The listing builds one solid part. Answer for the finished solid, in the listing's coordinates (mm). A direction names the side the tool comes from. Round coordinates to 2 decimals unless told otherwise and drop trailing zeros. Loops run counter-clockwise (first coordinate to the right, second up) from the corner with the lowest first, then second, coordinate; pieces in that order, holes last. Notation, with made-up numbers: M 43,44 L 51,44 A20 ccw 51,67 Z; hole C 36,85 d2. An arc over 180 degrees is marked long. Put each result on its own line as item: value. Start each with the question number.
(1) Section B-B, the plane x = 3.75 is taken. Count the separate pieces of the cut face and the enclosed holes in it, then the cut area to 3 significant figures.
(2) Section C-C, the plane y = 10 is taken. Determine the outline of the cut face in (x, z) (3 decimals), then the cut area to 3 significant figures.
(3) Straight lines are drawn through the part: line 1 (Z direction, x = 7.25, y = 1.25); line 2 (X direction, y = 2, z = 6.5); line 3 (X direction, y = 8.75, z = -7). For each, find the intervals that lie inside material, in ascending order.
(4) Section D-D, the plane z = 17 is taken. Determine the outline of the cut face in (x, y).
(5) Determine the mould class of faces 3 (the face through (-1, 1.9, 23.8)), 4 (the face through (-2, 12.7, -3)), 5 (the face through (-7, 2.1, -28.8)) for opening direction Z: released by +Z, released by -Z, zero draft, split by the parting line, or undercut.
(6) Which of the six approach directions +Z, -Z, +X, -X, +Y, -Y give full straight-line access (tool end or side, diameter ignored) to faces 1 (the face through (0.117, 1.932, -23.993)), 2 (the face through (-5.334, 1.878, 0.016))?
(7) Section A-A, the plane z = 0 is taken. Determine the outline of the cut face in (x, y) (3 decimals), then the cut area to 3 significant figures.
(8) Flat-ended cylindrical pins translate along their axes: P1, Ø6, axis at x = -4.91, z = -4.91, coming from the -Y side; P2, Ø7, axis at x = -4.91, z = 4.91, coming from the +Y side; P3, Ø8, axis at x = 4, z = 20.5, coming from the +Y side; P4, Ø8, axis at x = 3.5, z = -27.5, coming from the +Y side. Find the tip coordinate at first contact, or state that the pin passes through.
```python
from build123d import *

# Parameters (mm, degrees)
SKETCH1_W               = 20
SKETCH1_H               = 63.5
BOSS_EXTRUDE1_DEPTH     = 12.7
SKETCH2_R               = 3.175
SKETCH2_R_2             = 2.1844
CUT_EXTRUDE1_DEPTH      = 36.62797356
CUT_EXTRUDE2_DEPTH      = 36.62797356
CUT_EXTRUDE2_DEPTH_BACK = 36.62797356
SKETCH4_R               = 3.81
CUT_EXTRUDE3_DEPTH      = 8.89
SKETCH4_3_R             = 3.81
SKETCH4_3_R_2           = 2.1844
SKETCH4_3_R_3           = 5.334
SKETCH4_3_R_4           = 3.175
CUT_EXTRUDE4_DEPTH      = 3.81
SKETCH6_R               = 5.08
SKETCH6_R_2             = 2.667
CUT_EXTRUDE5_DEPTH      = 8.89
SKETCH6_4_R             = 2.667
CUT_EXTRUDE6_DEPTH      = 35.454239272
FILLET1_R               = 10.16


with BuildPart() as part:
    # Sketch1 → Boss-Extrude1 (new body)
    with BuildSketch(Plane(origin=(0, 0, 0), x_dir=(1, 0, 0), z_dir=(0, 1, 0))):
        Rectangle(SKETCH1_W, SKETCH1_H)
    extrude(amount=BOSS_EXTRUDE1_DEPTH)

    # Sketch2 → Cut-Extrude1 (cut, through all)
    with BuildSketch(Plane(origin=(0, 12.7, 0), x_dir=(1, 0, 0), z_dir=(0, 1, 0))):
        with Locations(Location((0, 0, 0), (0, 0, 270))):
            Circle(SKETCH2_R)
        with Locations(Location((-4.912200098, 4.912200098, 0), (0, 0, 270))):
            Circle(SKETCH2_R_2)
        with Locations(Location((4.912200098, -4.912200098, 0), (0, 0, 270))):
            Circle(SKETCH2_R_2)
        with Locations(Location((4.912200098, 4.912200098, 0), (0, 0, 90))):
            Circle(SKETCH2_R_2)
        with Locations(Location((-4.912200098, -4.912200098, 0), (0, 0, 90))):
            Circle(SKETCH2_R_2)
    extrude(amount=-CUT_EXTRUDE1_DEPTH, mode=Mode.SUBTRACT)

    # Sketch3 → Cut-Extrude2 (cut, two sides: drawn at the far end of the back side and taken through both)
    with BuildSketch(Plane(origin=(0, 0, 0), x_dir=(0, 0, -1), z_dir=(1, 0, 0)).offset(-CUT_EXTRUDE2_DEPTH_BACK)):
        with BuildLine():
            Line((31.75, 3.81), (31.75, 12.7))
            Line((31.75, 12.7), (10.906600098, 12.7))
            ThreePointArc((10.906600098, 12.7), (16.898665682, 6.209564949), (25.4, 3.81))
            Line((25.4, 3.81), (31.75, 3.81))
        make_face()
        with BuildLine():
            ThreePointArc((-25.4, 3.81), (-16.898665682, 6.209564949), (-10.906600098, 12.7))
            Line((-10.906600098, 12.7), (-31.75, 12.7))
            Line((-31.75, 12.7), (-31.75, 3.81))
            Line((-31.75, 3.81), (-25.4, 3.81))
        make_face()
    extrude(amount=CUT_EXTRUDE2_DEPTH + CUT_EXTRUDE2_DEPTH_BACK, mode=Mode.SUBTRACT)

    # Sketch4 → Cut-Extrude3 (cut)
    with BuildSketch(Plane.XZ):
        with Locations((-4.912200098, -4.912200098)):
            Circle(SKETCH4_R)
        with Locations((4.912200098, 4.912200098)):
            Circle(SKETCH4_R)
        with Locations((-4.912200098, 4.912200098)):
            Circle(SKETCH4_R)
        with Locations((4.912200098, -4.912200098)):
            Circle(SKETCH4_R)
    extrude(amount=-CUT_EXTRUDE3_DEPTH, mode=Mode.SUBTRACT)

    # Sketch4<3> → Cut-Extrude4 (cut)
    # profile 1 of 28: a face of its own
    with BuildSketch(Plane.XZ):
        with Locations((-4.912200098, 4.912200098)):
            Circle(SKETCH4_3_R)
        with Locations(Location((-4.912200098, 4.912200098, 0), (0, 0, 270))):
            Circle(SKETCH4_3_R_2, mode=Mode.SUBTRACT)
    # profile 2 of 28: a face of its own
    with BuildSketch(Plane.XZ):
        Circle(SKETCH4_3_R_3)
        with Locations(Location((0, 0, 0), (0, 0, 90))):
            Circle(SKETCH4_3_R_4, mode=Mode.SUBTRACT)
    # profile 3 of 28: a face of its own
    with BuildSketch(Plane.XZ):
        Circle(SKETCH4_3_R_3)
    # profile 4 of 28: a face of its own
    with BuildSketch(Plane.XZ):
        with Locations(Location((-4.912200098, 4.912200098, 0), (0, 0, 270))):
            Circle(SKETCH4_3_R_2)
    # profile 5 of 28: a face of its own
    with BuildSketch(Plane.XZ):
        with Locations((-4.912200098, 4.912200098)):
            Circle(SKETCH4_3_R)
    # profile 6 of 28: a face of its own
    with BuildSketch(Plane.XZ):
        Circle(SKETCH4_3_R_3)
        with Locations(Location((0, 0, 0), (0, 0, 90))):
            Circle(SKETCH4_3_R_4, mode=Mode.SUBTRACT)
    # profile 7 of 28: a face of its own
    with BuildSketch(Plane.XZ):
        with Locations((-4.912200098, -4.912200098)):
            Circle(SKETCH4_3_R)
    # profile 8 of 28: a face of its own
    with BuildSketch(Plane.XZ):
        Circle(SKETCH4_3_R_3)
        with Locations(Location((0, 0, 0), (0, 0, 90))):
            Circle(SKETCH4_3_R_4, mode=Mode.SUBTRACT)
    # profile 9 of 28: a face of its own
    with BuildSketch(Plane.XZ):
        with Locations((-4.912200098, -4.912200098)):
            Circle(SKETCH4_3_R)
        with Locations(Location((-4.912200098, -4.912200098, 0), (0, 0, 90))):
            Circle(SKETCH4_3_R_2, mode=Mode.SUBTRACT)
    # profile 10 of 28: a face of its own
    with BuildSketch(Plane.XZ):
        Circle(SKETCH4_3_R_3)
    # profile 11 of 28: a face of its own
    with BuildSketch(Plane.XZ):
        with Locations(Location((-4.912200098, -4.912200098, 0), (0, 0, 90))):
            Circle(SKETCH4_3_R_2)
    # profile 12 of 28: a face of its own
    with BuildSketch(Plane.XZ):
        with BuildLine():
            ThreePointArc((1.973854475, -2.486870224), (1.04518229, -2.998035854), (0, -3.175))
            Line((0, -3.175), (0, -5.334))
            ThreePointArc((0, -5.334), (0.560277089, -5.304492962), (1.114355409, -5.216298306))
            ThreePointArc((1.114355409, -5.216298306), (1.278123958, -3.767826643), (1.973854475, -2.486870224))
        make_face()
    # profile 13 of 28: a face of its own
    with BuildSketch(Plane.XZ):
        with BuildLine():
            Line((0, -5.334), (0, -3.175))
            ThreePointArc((0, -3.175), (-1.04518229, -2.998035854), (-1.973854475, -2.486870224))
            ThreePointArc((-1.973854475, -2.486870224), (-1.326729639, -3.623595587), (-1.102200098, -4.912200098))
            ThreePointArc((-1.102200098, -4.912200098), (-1.105240139, -5.064370621), (-1.114355409, -5.216298306))
            ThreePointArc((-1.114355409, -5.216298306), (-0.560277089, -5.304492962), (0, -5.334))
        make_face()
    # profile 14 of 28: a face of its own
    with BuildSketch(Plane.XZ):
        with Locations((4.912200098, -4.912200098)):
            Circle(SKETCH4_3_R)
        with Locations(Location((4.912200098, -4.912200098, 0), (0, 0, 270))):
            Circle(SKETCH4_3_R_2, mode=Mode.SUBTRACT)
    # profile 15 of 28: a face of its own
    with BuildSketch(Plane.XZ):
        Circle(SKETCH4_3_R_3)
        with Locations(Location((0, 0, 0), (0, 0, 90))):
            Circle(SKETCH4_3_R_4, mode=Mode.SUBTRACT)
    # profile 16 of 28: a face of its own
    with BuildSketch(Plane.XZ):
        Circle(SKETCH4_3_R_3)
    # profile 17 of 28: a face of its own
    with BuildSketch(Plane.XZ):
        with Locations(Location((4.912200098, -4.912200098, 0), (0, 0, 270))):
            Circle(SKETCH4_3_R_2)
    # profile 18 of 28: a face of its own
    with BuildSketch(Plane.XZ):
        with Locations((4.912200098, -4.912200098)):
            Circle(SKETCH4_3_R)
    # profile 19 of 28: a face of its own
    with BuildSketch(Plane.XZ):
        Circle(SKETCH4_3_R_3)
        with Locations(Location((0, 0, 0), (0, 0, 90))):
            Circle(SKETCH4_3_R_4, mode=Mode.SUBTRACT)
    # profile 20 of 28: a face of its own
    with BuildSketch(Plane.XZ):
        with Locations((4.912200098, 4.912200098)):
            Circle(SKETCH4_3_R)
    # profile 21 of 28: a face of its own
    with BuildSketch(Plane.XZ):
        Circle(SKETCH4_3_R_3)
        with Locations(Location((0, 0, 0), (0, 0, 90))):
            Circle(SKETCH4_3_R_4, mode=Mode.SUBTRACT)
    # profile 22 of 28: a face of its own
    with BuildSketch(Plane.XZ):
        with Locations((4.912200098, 4.912200098)):
            Circle(SKETCH4_3_R)
        with Locations(Location((4.912200098, 4.912200098, 0), (0, 0, 90))):
            Circle(SKETCH4_3_R_2, mode=Mode.SUBTRACT)
    # profile 23 of 28: a face of its own
    with BuildSketch(Plane.XZ):
        Circle(SKETCH4_3_R_3)
    # profile 24 of 28: a face of its own
    with BuildSketch(Plane.XZ):
        with Locations(Location((4.912200098, 4.912200098, 0), (0, 0, 90))):
            Circle(SKETCH4_3_R_2)
    # profile 25 of 28: a face of its own
    with BuildSketch(Plane.XZ):
        with BuildLine():
            Line((0, 3.175), (0, 5.334))
            ThreePointArc((0, 5.334), (-0.560277089, 5.304492962), (-1.114355409, 5.216298306))
            ThreePointArc((-1.114355409, 5.216298306), (-1.105240139, 5.064370621), (-1.102200098, 4.912200098))
            ThreePointArc((-1.102200098, 4.912200098), (-1.326729639, 3.623595587), (-1.973854475, 2.486870224))
            ThreePointArc((-1.973854475, 2.486870224), (-1.04518229, 2.998035854), (0, 3.175))
        make_face()
    # profile 26 of 28: a face of its own
    with BuildSketch(Plane.XZ):
        with BuildLine():
            ThreePointArc((1.114355409, 5.216298306), (0.560277089, 5.304492962), (0, 5.334))
            Line((0, 5.334), (0, 3.175))
            ThreePointArc((0, 3.175), (1.04518229, 2.998035854), (1.973854475, 2.486870224))
            ThreePointArc((1.973854475, 2.486870224), (1.278123958, 3.767826643), (1.114355409, 5.216298306))
        make_face()
    # profile 27 of 28: a face of its own
    with BuildSketch(Plane.XZ):
        with BuildLine():
            ThreePointArc((1.973854475, 2.486870224), (1.04518229, 2.998035854), (0, 3.175))
            Line((0, 3.175), (0, -3.175))
            ThreePointArc((0, -3.175), (1.04518229, -2.998035854), (1.973854475, -2.486870224))
            ThreePointArc((1.973854475, -2.486870224), (2.218123262, -2.218123262), (2.486870224, -1.973854475))
            ThreePointArc((2.486870224, -1.973854475), (2.998035854, -1.04518229), (3.175, 0))
            ThreePointArc((3.175, 0), (2.998035854, 1.04518229), (2.486870224, 1.973854475))
            ThreePointArc((2.486870224, 1.973854475), (2.218123262, 2.218123262), (1.973854475, 2.486870224))
        make_face()
    # profile 28 of 28: a face of its own
    with BuildSketch(Plane.XZ):
        with BuildLine():
            Line((0, -3.175), (0, 3.175))
            ThreePointArc((0, 3.175), (-1.04518229, 2.998035854), (-1.973854475, 2.486870224))
            ThreePointArc((-1.973854475, 2.486870224), (-2.218123262, 2.218123262), (-2.486870224, 1.973854475))
            ThreePointArc((-2.486870224, 1.973854475), (-3.175, 0), (-2.486870224, -1.973854475))
            ThreePointArc((-2.486870224, -1.973854475), (-2.218123262, -2.218123262), (-1.973854475, -2.486870224))
            ThreePointArc((-1.973854475, -2.486870224), (-1.04518229, -2.998035854), (0, -3.175))
        make_face()
    extrude(amount=-CUT_EXTRUDE4_DEPTH, mode=Mode.SUBTRACT)

    # Sketch6 → Cut-Extrude5 (cut)
    # profile 1 of 3: a face of its own
    with BuildSketch(Plane(origin=(0, 3.81, 0), x_dir=(1, 0, 0), z_dir=(0, 1, 0))):
        with Locations((0, -21.328300049)):
            Circle(SKETCH6_R)
        with Locations((0, -21.328300049)):
            Circle(SKETCH6_R_2, mode=Mode.SUBTRACT)
    # profile 2 of 3: a face of its own
    with BuildSketch(Plane(origin=(0, 3.81, 0), x_dir=(1, 0, 0), z_dir=(0, 1, 0))):
        with Locations((0, -21.328300049)):
            Circle(SKETCH6_R_2)
    # profile 3 of 3: a face of its own
    with BuildSketch(Plane(origin=(0, 3.81, 0), x_dir=(1, 0, 0), z_dir=(0, 1, 0))):
        with Locations((0, 21.328300049)):
            Circle(SKETCH6_R)
    extrude(amount=CUT_EXTRUDE5_DEPTH, mode=Mode.SUBTRACT)

    # Sketch6<4> → Cut-Extrude6 (cut, through all)
    with BuildSketch(Plane(origin=(0, 3.81, 0), x_dir=(1, 0, 0), z_dir=(0, 1, 0))):
        with Locations(Location((0, 21.328300049, 0), (0, 0, 270))):
            Circle(SKETCH6_4_R)
        with Locations(Location((0, -21.328300049, 0), (0, 0, 270))):
            Circle(SKETCH6_4_R)
    extrude(amount=-CUT_EXTRUDE6_DEPTH, mode=Mode.SUBTRACT)

    # Fillet1
    # the kernel refuses this fillet: 10.16 mm, written as the material it takes off along each edge
    with BuildSketch(Plane(origin=(10, -25.4, 31.75), x_dir=(0, 0, -1), z_dir=(0, 1, 0)), Plane(origin=(10, -25.4, -31.75), x_dir=(-1, 0, 0), z_dir=(0, 1, 0))) as fillet1_piece_1:
        with BuildLine():
            CenterArc((FILLET1_R, FILLET1_R), FILLET1_R, 180, 90)
            Line((0, FILLET1_R), (0, 0))
            Line((0, 0), (FILLET1_R, 0))
        make_face()
    extrude(amount=54.61, mode=Mode.SUBTRACT)
    with BuildSketch(Plane(origin=(-10, -25.4, 31.75), x_dir=(0, 0, -1), z_dir=(0, 1, 0)), Plane(origin=(-10, -25.4, -31.75), x_dir=(1, 0, 0), z_dir=(0, 1, 0))) as fillet1_piece_2:
        with BuildLine():
            CenterArc((FILLET1_R, -FILLET1_R), FILLET1_R, 90, 90)
            Line((0, -FILLET1_R), (0, 0))
            Line((0, 0), (FILLET1_R, 0))
        make_face()
    extrude(amount=54.61, mode=Mode.SUBTRACT)


solid = part.part
```
Recorded:
1. separate pieces: 3
1. enclosed holes: 0
1. area: 328 mm²
2. outline: M -10,-12.634 L 10,-12.634 L 10,12.634 L -10,12.634 Z; hole C -4.912,-4.912 d4.369; hole C -4.912,4.912 d4.369; hole C 0,0 d6.35; hole C 4.912,-4.912 d4.369; hole C 4.912,4.912 d4.369
2. area: 414 mm²
3. line 1: z = -28.54 to -7.92, -1.9 to 1.9, 7.92 to 28.54
3. line 2: x = -10 to -8.38, -1.45 to 1.45, 8.38 to 10
3. line 3: x = -10 to -8.1, -1.73 to 1.73, 8.1 to 10
4. outline: M -10,0 L 10,0 L 10,6.15 L 2.66,6.15 L 2.66,3.81 L -2.66,3.81 L -2.66,6.15 L -10,6.15 Z
5. face 3: undercut
5. face 4: zero draft
5. face 5: released by -Z
6. face 1: +Y, -Y
6. face 2: -Y
7. outline: M -10,0 L -5.334,0 L -5.334,3.81 L -3.175,3.81 L -3.175,12.7 L -10,12.7 Z; M 3.175,3.81 L 5.334,3.81 L 5.334,0 L 10,0 L 10,12.7 L 3.175,12.7 Z
7. area: 157 mm²
8. P1: stops at y = 8.89
8. P2: stops at y = 12.7
8. P3: stops at y = 6.46
8. P4: stops at y = 3.91
